For this review, take the finished solid that the model builds, in its own axes (mm). A direction names the side the tool comes from. Give positions to 0.01 mm unless a question says otherwise; leave off trailing zeros. Loops run counter-clockwise (first coordinate to the right, second up) from the corner with the lowest first, then second, coordinate; pieces in that order, holes last. Notation, with made-up numbers: (2, 55) -> (12, 55) arc R19 cw to (12, 85) -> close; hole circle Ø5 at (-28.75, 21). An arc over 180 degrees is marked (long way). Answer as CSV lines item,"result". Start each with the question number.
Item 1: Add section C-C on x = 111. State the section outline as (y, z) points.
Item 2: Machinability: for faces 1 (the face through (317, -275, 228)), 2 (the face through (-125, 330, 351)), 3 (the face through (725, 321, 376)), which of the approach directions +Z, -Z, +X, -X, +Y, -Y give a long, thin tool a straight path to every point of the face, cutting with its end or side? Answer none if there is none.
Item 3: Clearance check with a flat-ended pin moving along its axis: P1, Ø2, axis at x = 690, y = 222, coming from the +Z side. State where the tip first meets the part, or that it passes through.
Item 4: For L1, parallel to Y at x = 54, z = 390; L2, parallel to Y at x = 642, z = 408.5; L3, parallel to X at y = 651, z = 283, list the stretches that pass through material, from the lowest coordinate up. Write a range as from..to.
Item 5: Add section B-B on z = 375. State the section outline as (x, y) points.
Item 6: Add section D-D on z = 196. State the section outline as (x, y) points.
Item 7: Add section A-A on y = 229. State the section outline as (x, z) points.
Item 8: The part is to be moulded in two halves that separate along X. For faces 4 (the face through (-275, 333, 228)), 5 (the face through (317, 875, 222)), 6 (the face through (-83, 333, 475)), say which applies: +X half, -X half, draft (parallel to the pull), parting line (faces both ways), or undercut.
```python
from build123d import *

# Parameters (mm, degrees)
F0_W      = 1200
F0_H      = 1200
F0_W_2    = 1100
F0_H_2    = 1100
F1_DEPTH  = 450
F2_W      = 1200
F2_H      = 1200
F2_W_2    = 1100
F2_H_2    = 1100
F3_DEPTH  = 25
F4_W      = 900
F4_H      = 700
F5_DEPTH  = 200
F6_W      = 1200
F6_H      = 1200
F6_W_2    = 1100
F6_H_2    = 1100
F7_DEPTH  = 25
F8_W      = 800
F8_H      = 600
F9_DEPTH  = 200
F10_R     = 50
F11_DEPTH = 50
F12_R     = 62.5
F12_R_2   = 50
F13_DEPTH = 25


with BuildPart() as f1:
    # F0 (on Top) → F1 (new body)
    with BuildSketch(Plane.XY):
        with Locations((325, 325)):
            Rectangle(F0_W, F0_H)
        with Locations((325, 325)):
            Rectangle(F0_W_2, F0_H_2, mode=Mode.SUBTRACT)
    extrude(amount=F1_DEPTH)

    # F2 (on face) → F3 (join)
    with BuildSketch(Plane.XY.offset(450)):
        with Locations((325, 325)):
            Rectangle(F2_W, F2_H)
        with Locations((325, 325)):
            Rectangle(F2_W_2, F2_H_2, mode=Mode.SUBTRACT)
        with Locations((325, 325)):
            Rectangle(F2_W_2, F2_H_2)
    extrude(amount=F3_DEPTH)

    # F4 (on face) → F5 (join)
    with BuildSketch(Plane(origin=(0, 0, 450), x_dir=(1, 0, 0), z_dir=(0, 0, -1))):
        with Locations((325, -325)):
            Rectangle(F4_W, F4_H)
    extrude(amount=F5_DEPTH)

    # F6 (on face) → F7 (join)
    with BuildSketch(Plane(origin=(0, 0, 0), x_dir=(1, 0, 0), z_dir=(0, 0, -1))):
        with Locations((325, -325)):
            Rectangle(F6_W, F6_H)
        with Locations((325, -325)):
            Rectangle(F6_W_2, F6_H_2, mode=Mode.SUBTRACT)
        with Locations((325, -325)):
            Rectangle(F6_W_2, F6_H_2)
    extrude(amount=F7_DEPTH)

    # F8 (on face) → F9 (cut)
    with BuildSketch(Plane.XY.offset(475)):
        with Locations((325, 325)):
            Rectangle(F8_W, F8_H)
    extrude(amount=-F9_DEPTH, mode=Mode.SUBTRACT)

    # F10 (on face) → F11 (cut, through all)
    with BuildSketch(Plane.XZ.offset(-625)):
        with Locations((589.7976160049, 375)):
            Circle(F10_R)
    extrude(amount=-F11_DEPTH, mode=Mode.SUBTRACT)

    # F12 (on face) → F13 (join)
    with BuildSketch(Plane.XZ.offset(-625)):
        with Locations((589.7976160049, 375)):
            Circle(F12_R)
        with Locations((589.7976160049, 375)):
            Circle(F12_R_2, mode=Mode.SUBTRACT)
        with Locations((589.7976160049, 375)):
            Circle(F12_R_2)
    extrude(amount=F13_DEPTH)


solid = f1.part
```
Computed values:
1,outline,"(-275, -25) -> (925, -25) -> (925, 475) -> (625, 475) -> (625, 275) -> (25, 275) -> (25, 475) -> (-275, 475) -> close; hole (-225, 0) -> (875, 0) -> (875, 450) -> (675, 450) -> (675, 250) -> (-25, 250) -> (-25, 450) -> (-225, 450) -> close"
2,face 1,"+Z, -Z, +X, -X, -Y"
2,face 2,"none"
2,face 3,"+Z"
3,P1,"z = 275"
4,L1,"-275..-225, -25..25, 625..675, 875..925"
4,L2,"-275..-225, -25..25, 600..675, 875..925"
4,L3,"-275..-225, -125..775, 875..925"
5,outline,"(-275, -275) -> (925, -275) -> (925, 925) -> (-275, 925) -> close; (-125, -25) -> (775, -25) -> (775, 675) -> (639.8, 675) -> (639.8, 625) -> (539.8, 625) -> (539.8, 675) -> (-125, 675) -> close; hole (-225, -225) -> (875, -225) -> (875, 875) -> (-225, 875) -> close; hole (-75, 25) -> (725, 25) -> (725, 625) -> (652.3, 625) -> (652.3, 600) -> (527.3, 600) -> (527.3, 625) -> (-75, 625) -> close"
6,outline,"(-275, -275) -> (925, -275) -> (925, 925) -> (-275, 925) -> close; hole (-225, -225) -> (875, -225) -> (875, 875) -> (-225, 875) -> close"
7,outline,"(-275, -25) -> (925, -25) -> (925, 475) -> (725, 475) -> (725, 275) -> (-75, 275) -> (-75, 475) -> (-275, 475) -> close; hole (-225, 0) -> (875, 0) -> (875, 450) -> (775, 450) -> (775, 250) -> (-125, 250) -> (-125, 450) -> (-225, 450) -> close"
8,face 4,"-X half"
8,face 5,"undercut"
8,face 6,"draft"
